```python
from build123d import *

# Parameters (mm, degrees)
F0_W      = 250
F0_H      = 250
F1_DEPTH  = 600
F2_DEPTH  = 500
F3_DEPTH  = 400
F4_DEPTH  = 300
F5_W      = 200
F5_H      = 200
F6_DEPTH  = 575
F7_W      = 200
F7_H      = 200
F8_DEPTH  = 475
F9_W      = 200
F9_H      = 200
F10_DEPTH = 375
F11_W     = 200
F11_H     = 200
F12_DEPTH = 275


with BuildPart() as f1:
    # F0 (on Top) → F1 (new body)
    with BuildSketch(Plane.XY):
        with Locations((125, 375)):
            Rectangle(F0_W, F0_H)
    extrude(amount=F1_DEPTH)

    # F0 (on Top) → F2 (join)
    with BuildSketch(Plane.XY):
        with Locations((375, 375)):
            Rectangle(F0_W, F0_H)
    extrude(amount=F2_DEPTH)

    # F0 (on Top) → F3 (join)
    with BuildSketch(Plane.XY):
        with Locations((375, 125)):
            Rectangle(F0_W, F0_H)
    extrude(amount=F3_DEPTH)

    # F0 (on Top) → F4 (join)
    with BuildSketch(Plane.XY):
        with Locations((125, 125)):
            Rectangle(F0_W, F0_H)
    extrude(amount=F4_DEPTH)

    # F5 (on face) → F6 (cut)
    with BuildSketch(Plane.XY.offset(600)):
        with Locations((125, 375)):
            Rectangle(F5_W, F5_H)
    extrude(amount=-F6_DEPTH, mode=Mode.SUBTRACT)

    # F7 (on face) → F8 (cut)
    with BuildSketch(Plane.XY.offset(500)):
        with Locations((375, 375)):
            Rectangle(F7_W, F7_H)
    extrude(amount=-F8_DEPTH, mode=Mode.SUBTRACT)

    # F9 (on face) → F10 (cut)
    with BuildSketch(Plane.XY.offset(400)):
        with Locations((375, 125)):
            Rectangle(F9_W, F9_H)
    extrude(amount=-F10_DEPTH, mode=Mode.SUBTRACT)

    # F11 (on face) → F12 (cut)
    with BuildSketch(Plane.XY.offset(300)):
        with Locations((125, 125)):
            Rectangle(F11_W, F11_H)
    extrude(amount=-F12_DEPTH, mode=Mode.SUBTRACT)


solid = f1.part
```
Source: CAD feature listing. Evaluate the final solid. Frame: model axes, mm. A direction names the side the tool comes from. Coordinates: 2 decimals unless noted, no trailing zeros. Loops run counter-clockwise (first coordinate to the right, second up) from the corner with the lowest first, then second, coordinate; pieces in that order, holes last. Notation, with made-up numbers: M 3,33 L 62,33 A24 ccw 62,68 Z; hole C -33,74 d5. An arc over 180 degrees is marked long. Use CSV: the item, a comma, the result in double quotes.
(1) Draft query along Y for faces 1 (the face through (247, 254, 0)), 2 (the face through (124, 376, 25)). Return one class per face: pulls with the +Y half, pulls with the -Y half, needs draft (parallel to the pull), parting line crosses it, or undercut.
Answers follow:
face 1,"needs draft"
face 2,"undercut"
(2) Cut plane C-C on z = 187. Return loops of the section in (x, y), and give its area (3 significant figures).
Answers follow:
outline,"M 0,0 L 500,0 L 500,500 L 0,500 Z; hole M 25,25 L 225,25 L 225,225 L 25,225 Z; hole M 25,275 L 225,275 L 225,475 L 25,475 Z; hole M 275,25 L 475,25 L 475,225 L 275,225 Z; hole M 275,275 L 475,275 L 475,475 L 275,475 Z"
area,"90,000 mm²"
(3) Contact query for flat-ended pins moving along their axis: pin 1 (6 mm diameter, centred on x = 56.5, z = 335.5, fed in from -Y); pin 2 (1.5 mm diameter, centred on x = 273, y = 366.5, fed in from +Z). Output: stop coordinate, or through.
Answers follow:
pin 1,"y = 250"
pin 2,"z = 500"
(4) Cut plane D-D on x = 65. Return loops of the section in (y, z).
Answers follow:
outline,"M 0,0 L 500,0 L 500,600 L 475,600 L 475,25 L 275,25 L 275,600 L 250,600 L 250,300 L 225,300 L 225,25 L 25,25 L 25,300 L 0,300 Z"
(5) Line query: line 1 (Y direction, x = 382.5, z = 35.5); line 2 (Y direction, x = 81.5, z = 567). Output: solid intervals per line, ascending. Write a range as [from, to].
Answers follow:
line 1,"[0, 25], [225, 275], [475, 500]"
line 2,"[250, 275], [475, 500]"
(6) Cut plane B-B on y = 52. Return loops of the section in (x, z), and give its area (3 significant figures).
Answers follow:
outline,"M 0,0 L 500,0 L 500,400 L 475,400 L 475,25 L 275,25 L 275,400 L 250,400 L 250,300 L 225,300 L 225,25 L 25,25 L 25,300 L 0,300 Z"
area,"45,000 mm²"
(7) Cut plane A-A on z = 343.5. Return loops of the section in (x, y).
Answers follow:
outline,"M 0,250 L 250,250 L 250,0 L 500,0 L 500,500 L 0,500 Z; hole M 25,275 L 225,275 L 225,475 L 25,475 Z; hole M 275,25 L 475,25 L 475,225 L 275,225 Z; hole M 275,275 L 475,275 L 475,475 L 275,475 Z"
(8) Reachability of faces 3 (the face through (25, 374, 317)), 4 (the face through (234, 127, 300)), 5 (the face through (250, 373, 549)), 6 (the face through (262, 127, 400)) from +Z, -Z, +X, -X, +Y, -Y: full face, straight path, thin tool, end or side. Return the list, or none.
Answers follow:
face 3,"+Z"
face 4,"+Z, -X, -Y"
face 5,"+Z, +X, +Y, -Y"
face 6,"+Z, +X, -X, -Y"
